Build history of the part. All positions in model axes, mm. A direction names the side the tool comes from. Give positions to 0.01 mm unless a question says otherwise; leave off trailing zeros. One line per item, written item: value. Start each with the question number.
from build123d import *

# Parameters (mm, degrees)
F0_W     = 8.5
F0_H     = 20
F2_ANGLE = -180
F3_DEPTH = 65
F5_R     = 1
F6_DEPTH = 28


with BuildPart() as f2:
    # F0 (on Top) → F2 (revolve)
    with BuildSketch(Plane.XY):
        with BuildLine():
            Line((0, 95), (0, 65))
            Line((0, 65), (5.5, 65))
            Line((5.5, 65), (5.5, 20))
            Line((5.5, 20), (14, 20))
            Line((14, 20), (16, 20))
            add(Edge.make_bspline(
                [(0, 95), (11.437606, 95.100096), (16.261564, 47.378998), (16, 20)],
                knots=[0, 0, 0, 0, 76.687678, 76.687678, 76.687678, 76.687678], degree=3))
        make_face()
        with Locations((9.75, 10)):
            Rectangle(F0_W, F0_H)
    revolve(axis=Axis((0, 57.5, 0), (0, 1, 0)), revolution_arc=F2_ANGLE)

    # F1 (on Front) → F3 (cut)
    with BuildSketch(Plane.XZ):
        with BuildLine():
            Line((0, 5.5), (0, 0))
            ThreePointArc((0, 0), (3.889087, 1.610913), (5.5, 5.5))
            Line((5.5, 5.5), (0, 5.5))
        make_face()
        with BuildLine():
            ThreePointArc((5.5, 5.5), (3.889087, 1.610913), (0, 0))
            Line((0, 0), (5.5, 0))
            Line((5.5, 0), (5.5, 5.5))
        make_face()
        with BuildLine():
            Line((-5.5, 0), (0, 0))
            ThreePointArc((0, 0), (-3.889087, 1.610913), (-5.5, 5.5))
            Line((-5.5, 5.5), (-5.5, 0))
        make_face()
        with BuildLine():
            ThreePointArc((-5.5, 5.5), (-3.889087, 1.610913), (0, 0))
            Line((0, 0), (0, 5.5))
            Line((0, 5.5), (-5.5, 5.5))
        make_face()
        with BuildLine():
            Line((-5.5, 5.5), (0, 5.5))
            Line((0, 5.5), (0, 11))
            ThreePointArc((0, 11), (-3.889087, 9.389087), (-5.5, 5.5))
        make_face()
        with BuildLine():
            Line((0, 11), (0, 5.5))
            Line((0, 5.5), (5.5, 5.5))
            ThreePointArc((5.5, 5.5), (3.889087, 9.389087), (0, 11))
        make_face()
    extrude(amount=-F3_DEPTH, mode=Mode.SUBTRACT)

    # F5 (on offset) → F6 (cut)
    with BuildSketch(Plane.YZ.offset(14)):
        with Locations((10, 0.00426)):
            Circle(F5_R)
    extrude(amount=-F6_DEPTH, mode=Mode.SUBTRACT)


solid = f2.part
1) Tool access for faces 1 (the flat face through (-10, 5, 0)), 2 (the cylindrical face through (0, 10, 14)), 3 (the flat face through (-5.5, 32, 3)): list every direction of +Z, -Z, +X, -X, +Y, -Y with a clear straight run to the whole face (end or side of a thin tool).
2) Drop flat-ended pins along their axis: P1, Ø4.5, axis at y = 36.5, z = 2.5, coming from the +X side; P2, Ø8, axis at y = 73.5, z = 12.5, coming from the +X side; P3, Ø4.5, axis at y = 46, z = 3.5, coming from the -X side. Give the stop position or say it passes through.
3) Drill centre lines: line 1 (X direction, y = 49.5, z = 3.5); line 2 (X direction, y = 38, z = 9); line 3 (Z direction, x = 2, y = 84). Where is each one in solid material? Low to high.
4) Pull direction Y, two halves, no side cores. Call faces 4 (the cylindrical face through (-9.691, 10.022, 1.004)), 5 (the flat face through (0, 65, 6)), 6 (the flat face through (10, 5, 0)): pulls with the +Y half, pulls with the -Y half, needs draft (parallel to the pull), parting line crosses it, or undercut.
Results list:
1. face 1: -Z, +X, -X, +Y, -Y
1. face 2: +Z, -Y
1. face 3: -Z, -Y
2. P1: stops at x = 15.68
2. P2: stops at x = 7.64
2. P3: stops at x = -15.02
3. line 1: x = -14.29 to -5.5, 5.5 to 14.29
3. line 2: x = -12.68 to -4.24, 4.24 to 12.68
3. line 3: z = 0 to 8.32
4. face 4: undercut
4. face 5: pulls with the -Y half
4. face 6: needs draft
